Input: dimensioned drawing with shaded views. Units: mm. Origin: part minimum x, y, z. A direction names the side the tool comes from. Coordinates: 2 decimals unless noted, no trailing zeros. Loops run counter-clockwise (first coordinate to the right, second up) from the corner with the lowest first, then second, coordinate; pieces in that order, holes last.
Item 1: Contact query for flat-ended pins moving along their axis: P1, Ø12, axis at y = 34, z = 52.5, coming from the +X side; P2, Ø1.5, axis at x = 37.5, y = 13, coming from the -Z side; P3, Ø3, axis at y = 51, z = 3, coming from the +X side. Output: stop coordinate, or through.
Item 2: Pull-direction query (Y, two-part tool) for the marked faces 1, 2 and 3; classes: released by +Y, released by -Y, zero draft, split by the parting line, or undercut.
Item 3: Section A-A on x = 20.5. Return loops of the section in (y, z), and give its area (3 significant figures).
Item 4: Ray query, line 1 along X through (y, z) = (7, 7.5); line 2 along Y through (x, z) = (22, 29); line 3 along X through (y, z) = (44.5, 41). Return the intervals inside material, ascending.
Item 5: Section B-B on y = 19.5. Return loops of the section in (x, z), and give its area (3 significant figures).
Item 6: Reachability of the marked faces 4, 5, 6 and 7 from +Z, -Z, +X, -X, +Y, -Y: full face, straight path, thin tool, end or side. Return the list, or none.
Item 7: Section C-C on z = 34. Return loops of the section in (x, y), and give its area (3 significant figures).
Item 8: Section D-D on y = 59. Return loops of the section in (x, z), and give its area (3 significant figures).
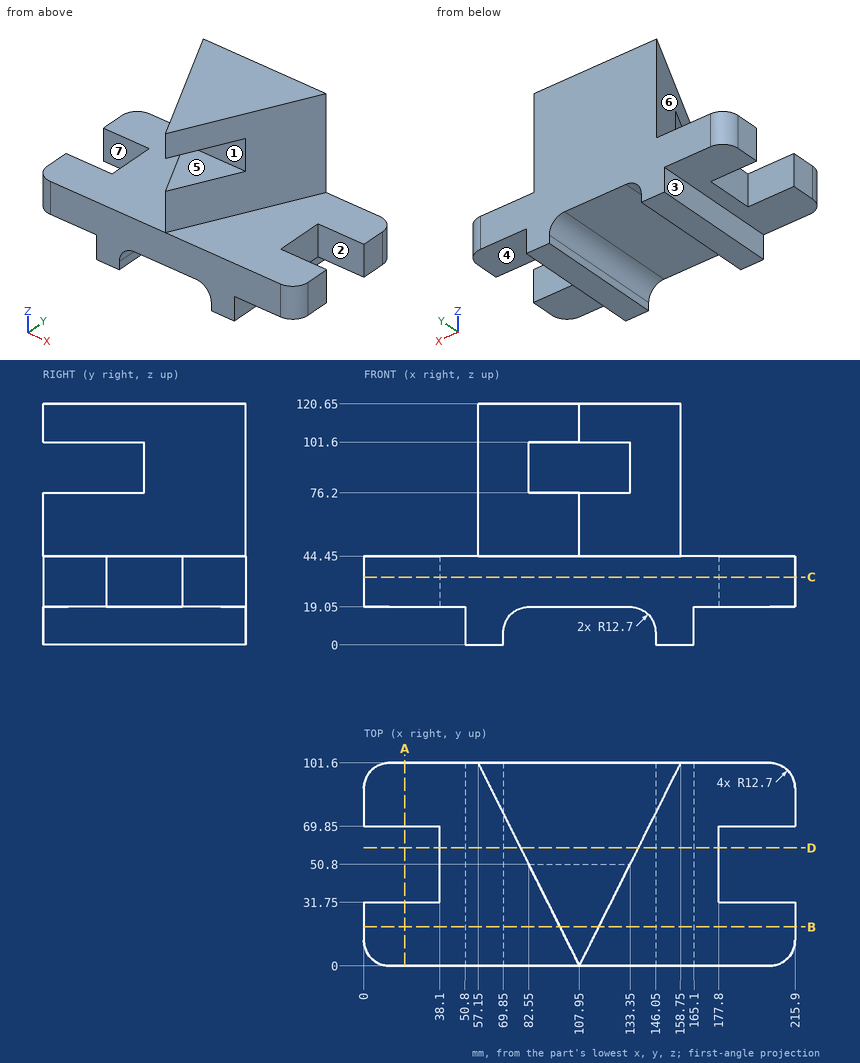
Results found:
1. P1: stops at x = 127.95
1. P2: stops at z = 19.05
1. P3: stops at x = 165.1
2. face 1: released by -Y
2. face 2: undercut
2. face 3: zero draft
3. outline: (0, 19.05) - (31.75, 19.05) - (31.75, 44.45) - (0, 44.45) - close; (69.85, 19.05) - (101.6, 19.05) - (101.6, 44.45) - (69.85, 44.45) - close
3. area: 1,610 mm2
4. line 1: x = 50.8 to 69.9, 146 to 165.1
4. line 2: y = 0 to 31.75, 69.85 to 101.6
4. line 3: x = 38.1 to 177.8
5. outline: (0, 19.05) - (50.8, 19.05) - (50.8, 0) - (69.85, 0) - (69.85, 6.35) arc R12.7 cw to (82.55, 19.05) - (133.35, 19.05) arc R12.7 cw to (146.05, 6.35) - (146.05, 0) - (165.1, 0) - (165.1, 19.05) - (215.9, 19.05) - (215.9, 44.45) - (117.7, 44.45) - (117.7, 76.2) - (98.2, 76.2) - (98.2, 44.45) - (0, 44.45) - close; (98.2, 101.6) - (117.7, 101.6) - (117.7, 120.65) - (98.2, 120.65) - close
5. area: 7,270 mm2
6. face 4: -Z, +X, +Y, -Y
6. face 5: +X, -X, -Y
6. face 6: +Z, -X, -Y
6. face 7: +Z, -Z, -X
7. outline: (0, 12.7) arc R12.7 ccw to (12.7, 0) - (203.2, 0) arc R12.7 ccw to (215.9, 12.7) - (215.9, 31.75) - (177.8, 31.75) - (177.8, 69.85) - (215.9, 69.85) - (215.9, 88.9) arc R12.7 ccw to (203.2, 101.6) - (12.7, 101.6) arc R12.7 ccw to (0, 88.9) - (0, 69.85) - (38.1, 69.85) - (38.1, 31.75) - (0, 31.75) - close
7. area: 18,900 mm2
8. outline: (38.1, 19.05) - (50.8, 19.05) - (50.8, 0) - (69.85, 0) - (69.85, 6.35) arc R12.7 cw to (82.55, 19.05) - (133.35, 19.05) arc R12.7 cw to (146.05, 6.35) - (146.05, 0) - (165.1, 0) - (165.1, 19.05) - (177.8, 19.05) - (177.8, 44.45) - (137.45, 44.45) - (137.45, 120.65) - (78.45, 120.65) - (78.45, 44.45) - (38.1, 44.45) - close
8. area: 8,840 mm2
